```python
from build123d import *

# Parameters (mm, degrees)
SKETCH1_R           = 4.9
BOSS_EXTRUDE1_DEPTH = 13.8
SKETCH2_R           = 6
BOSS_EXTRUDE2_DEPTH = 19.1
SKETCH7_R           = 2.625
CUT_EXTRUDE1_DEPTH  = 33.9
CHAMFER1_SIZE       = 0.4


with BuildPart() as part:
    # Sketch1 → Boss-Extrude1 (new body)
    with BuildSketch(Plane(origin=(0, 0, 0), x_dir=(1, 0, 0), z_dir=(0, 1, 0))):
        Circle(SKETCH1_R)
    extrude(amount=BOSS_EXTRUDE1_DEPTH)

    # Sketch2 → Boss-Extrude2 (add)
    with BuildSketch(Plane(origin=(0, 13.8, 0), x_dir=(1, 0, 0), z_dir=(0, 1, 0))):
        Circle(SKETCH2_R)
    extrude(amount=BOSS_EXTRUDE2_DEPTH)

    # Sketch7 → Cut-Extrude1 (cut, through all)
    with BuildSketch(Plane(origin=(0, 0, 0), x_dir=(1, 0, 0), z_dir=(0, 1, 0))):
        Circle(SKETCH7_R)
    extrude(amount=CUT_EXTRUDE1_DEPTH, mode=Mode.SUBTRACT)

    # Chamfer1
    chamfer1_edges = [part.edges().sort_by_distance(p)[0] for p in [
        (-2.625, 0, 0),
    ]]
    chamfer(chamfer1_edges, length=CHAMFER1_SIZE)


solid = part.part
```
The model under review builds one solid part; all positions refer to its coordinate system, in mm. A direction names the side the tool comes from. Give positions to 0.01 mm unless a question says otherwise; leave off trailing zeros. Write each loop counter-clockwise with the first axis right and the second up, starting at its lowest first coordinate (ties: lowest second). Pieces come first, ordered by that corner, then holes.
(1) Consider section C-C, the plane y = 5. Give the boundary of the cut face in (x, z) (3 decimals).
(2) Consider section B-B, the plane z = 0. Give the boundary of the cut face in (x, y) (3 decimals).
(3) Tool access review of faces 1 (the flat face through (1, 13.8, 5)), 2 (the flat face through (3, 32.9, 1)): name each direction out of +Z, -Z, +X, -X, +Y, -Y from which nothing blocks a thin tool from reaching the whole face with its end or side.
(4) To check wall thickness, follow L1, parallel to Z at x = 0, y = 19 (3 decimals); L2, parallel to Z at x = 0, y = 11.5 (3 decimals). State the ranges of each line that lie inside material, in increasing order.
(5) Consider section A-A, the plane x = 0. Give the boundary of the cut face in (y, z) (3 decimals), and give its area (3 significant figures).
(6) For P1, Ø2, axis at x = 1.5, y = 5.5, coming from the -Z side; P2, Ø3, axis at x = -4, y = 8, coming from the -Z side; P3, Ø5, axis at y = 20, z = 1, coming from the +X side; P4, Ø3, axis at x = -3, y = 17.5, coming from the +Z side, all flat-tipped, find the tip position at first contact; note any pin that passes through.
(7) The part is to be moulded in two halves that separate along Z. For faces 3 (the cylindrical face through (-6, 23, 0)), 4 (the flat face through (-0.1, 0, 3.2)), 5 (the cylindrical face through (2.5, 16.4, -0.8)), say which applies: released by +Z, released by -Z, zero draft, split by the parting line, or undercut.
(8) Consider section D-D, the plane z = -3.5. Give the boundary of the cut face in (x, y), and give its area (3 significant figures).
Returned:
1. outline: circle Ø9.8 at (0, 0); hole circle Ø5.25 at (0, 0)
2. outline: (-6, 13.8) - (-4.9, 13.8) - (-4.9, 0) - (-3.025, 0) - (-2.625, 0.4) - (-2.625, 32.9) - (-6, 32.9) - close; (2.625, 0.4) - (3.025, 0) - (4.9, 0) - (4.9, 13.8) - (6, 13.8) - (6, 32.9) - (2.625, 32.9) - close
3. face 1: -Y
3. face 2: +Z, -Z, +X, -X, +Y
4. L1: z = -6 to -2.625, 2.625 to 6
4. L2: z = -4.9 to -2.625, 2.625 to 4.9
5. outline: (0, -4.9) - (13.8, -4.9) - (13.8, -6) - (32.9, -6) - (32.9, -2.625) - (0.4, -2.625) - (0, -3.025) - close; (0, 3.025) - (0.4, 2.625) - (32.9, 2.625) - (32.9, 6) - (13.8, 6) - (13.8, 4.9) - (0, 4.9) - close
5. area: 192 mm2
6. P1: stops at z = -4.87
6. P2: stops at z = -4.21
6. P3: stops at x = 6
6. P4: stops at z = 5.81
7. face 3: split by the parting line
7. face 4: zero draft
7. face 5: undercut
8. outline: (-4.87, 13.8) - (-3.43, 13.8) - (-3.43, 0) - (3.43, 0) - (3.43, 13.8) - (4.87, 13.8) - (4.87, 32.9) - (-4.87, 32.9) - close
8. area: 281 mm2
